from build123d import *

# Parameters (mm, degrees)
SKETCH_W        = 45
SKETCH_H        = 43
PAD_DEPTH       = 65
SKETCH001_W     = 42
SKETCH001_H     = 42
POCKET_DEPTH    = 37
POCKET001_DEPTH = 43.001
SKETCH003_R     = 12
SKETCH003_R_2   = 1.5
POCKET002_DEPTH = 28.001
SKETCH004_R     = 6
POCKET003_DEPTH = 10
SKETCH005_W     = 62
SKETCH005_H     = 40
SKETCH005_R     = 2
PAD001_DEPTH    = 2
FILLET_R        = 2


with BuildPart() as part:
    # Sketch → Pad (new body)
    with BuildSketch(Plane.YZ):
        with Locations((22.5, 21.5)):
            Rectangle(SKETCH_W, SKETCH_H)
    extrude(amount=PAD_DEPTH)

    # Sketch001 (on Face6 of Pad) → Pocket (cut)
    with BuildSketch(Plane.YZ.offset(65)):
        with Locations((22.5, 21.5)):
            Rectangle(SKETCH001_W, SKETCH001_H)
    extrude(amount=-POCKET_DEPTH, mode=Mode.SUBTRACT)

    # Sketch002 (on Face6 of Pocket) → Pocket001 (cut, through all)
    with BuildSketch(Plane(origin=(0, 0, 43), x_dir=(0, -1, 0), z_dir=(0, 0, 1))):
        Polygon((-43.5, 65), (0, 28), (0, 65), align=None)
    extrude(amount=-POCKET001_DEPTH, mode=Mode.SUBTRACT)

    # Sketch003 (on Face12 of Pocket001) → Pocket002 (cut, through all)
    with BuildSketch(Plane.YZ.offset(28)):
        with Locations((22.5, 21.5)):
            Circle(SKETCH003_R)
        with Locations((7, 37)):
            Circle(SKETCH003_R_2)
        with Locations((38, 37)):
            Circle(SKETCH003_R_2)
        with Locations((7, 6)):
            Circle(SKETCH003_R_2)
        with Locations((38, 6)):
            Circle(SKETCH003_R_2)
    extrude(amount=-POCKET002_DEPTH, mode=Mode.SUBTRACT)

    # Sketch004 (on Face1 of Pocket002) → Pocket003 (cut)
    with BuildSketch(Plane.YX):
        with Locations((15, 10)):
            Circle(SKETCH004_R)
    extrude(amount=-POCKET003_DEPTH, mode=Mode.SUBTRACT)

    # Sketch005 (on Face4 of Pocket003) → Pad001 (join)
    with BuildSketch(Plane.ZX.offset(45)):
        with Locations((21.5, 45)):
            Rectangle(SKETCH005_W, SKETCH005_H)
        with Locations((-5.5, 60)):
            Circle(SKETCH005_R, mode=Mode.SUBTRACT)
        with Locations((-5.5, 45)):
            Circle(SKETCH005_R, mode=Mode.SUBTRACT)
        with Locations((-5.5, 30)):
            Circle(SKETCH005_R, mode=Mode.SUBTRACT)
        with Locations((48.5, 60)):
            Circle(SKETCH005_R, mode=Mode.SUBTRACT)
        with Locations((48.5, 45)):
            Circle(SKETCH005_R, mode=Mode.SUBTRACT)
        with Locations((48.5, 30)):
            Circle(SKETCH005_R, mode=Mode.SUBTRACT)
    extrude(amount=PAD001_DEPTH)

    # Fillet
    fillet_edges = [part.edges().sort_by_distance(p)[0] for p in [
        (65, 46, 52.5),
        (25, 46, 52.5),
        (65, 46, -9.5),
        (25, 46, -9.5),
    ]]
    fillet(fillet_edges, radius=FILLET_R)


solid = part.part
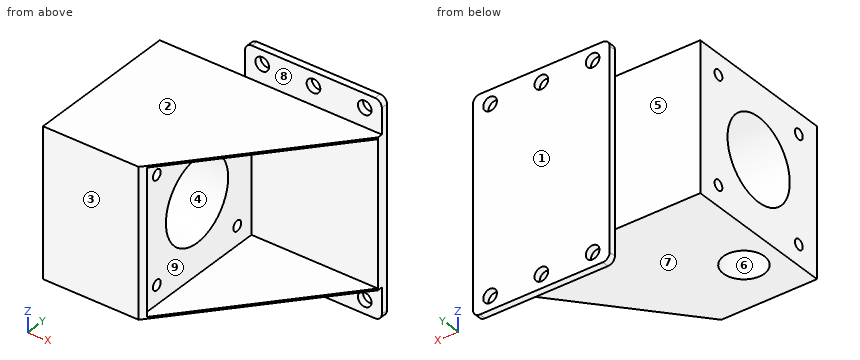
The listing builds one solid part. Answer for the finished solid, in the listing's coordinates (mm). Face numbers are marked on the shaded views. A direction names the side the tool comes from. Give positions to 0.01 mm unless a question says otherwise; leave off trailing zeros. Order: outer loops, then holes, each group sorted by start corner. A loop starts at its lowest first (then second) coordinate and runs counter-clockwise, first axis right, second up. Notation, with made-up numbers: (-11, 16.5) -> (12, 16.5) arc R19 cw to (12, 42.5) -> close; hole circle Ø9 at (70, 51). An arc over 180 degrees is marked (long way). Put each result on its own line as item: value.
Item 1: For a pull along Y with two mould halves and no side action, classify the marked faces 1, 2, 3 and 4 as released by +Y, released by -Y, zero draft, split by the parting line, or undercut.
Established:
face 1: released by +Y
face 2: zero draft
face 3: released by -Y
face 4: undercut
Item 2: Straight lines are drawn through the part: line 1 (Z direction, x = 6, y = 38); line 2 (X direction, y = 45.45, z = -5.5); line 3 (Y direction, x = 10, z = 8). For each, find the intervals that lie inside material, in ascending order.
Established:
line 1: z = 0 to 4.5, 7.5 to 35.5, 38.5 to 43
line 2: x = 25 to 28, 32 to 43, 47 to 58, 62 to 65
line 3: y = 0 to 9, 21 to 45
Item 3: Given P1, Ø2, axis at y = 46.5, z = 10, coming from the -X side; P2, Ø5, axis at y = 7, z = 37, coming from the +X side; P3, Ø5, axis at x = 39.5, z = -3.5, coming from the -Y side; P4, Ø2.5, axis at x = 30, z = 48.5, coming from the -Y side, each flat-ended and moving along its own axis, determine where each tip first touches the part or whether it passes through.
Established:
P1: stops at x = 25
P2: stops at x = 28
P3: stops at y = 45
P4: passes through
Item 4: A cutting plane is placed at A-A on z = 6. Give the vertices of the cut face in (x, y).
Established:
outline: (0, 0) -> (28, 0) -> (29.28, 1.5) -> (28, 1.5) -> (28, 5.5) -> (0, 5.5) -> close; (0, 8.5) -> (28, 8.5) -> (28, 36.5) -> (0, 36.5) -> close; (0, 39.5) -> (28, 39.5) -> (28, 43.5) -> (65, 43.5) -> (65, 47) -> (25, 47) -> (25, 45) -> (0, 45) -> close; hole circle Ø12 at (10, 15)
Item 5: A cutting plane is placed at C-C on z = 37. Give the vertices of the cut face in (x, y).
Established:
outline: (0, 0) -> (28, 0) -> (29.28, 1.5) -> (28, 1.5) -> (28, 5.5) -> (0, 5.5) -> close; (0, 8.5) -> (28, 8.5) -> (28, 36.5) -> (0, 36.5) -> close; (0, 39.5) -> (28, 39.5) -> (28, 43.5) -> (65, 43.5) -> (65, 47) -> (25, 47) -> (25, 45) -> (0, 45) -> close
Item 6: For the marked faces 5, 6, 7, 8 and 9, determine the directions among +Z, -Z, +X, -X, +Y, -Y from which every point of the face is accessible in a straight line to the end or side of a thin tool.
Established:
face 5: +Z, -Z, -X, +Y
face 6: -Z
face 7: -Z, +X, -X, -Y
face 8: +Z, +X, -X, -Y
face 9: +X
Item 7: A cutting plane is placed at D-D on y = 31.5. Give the vertices of the cut face in (x, z), plus the area to 3 significant figures.
Established:
outline: (0, 0) -> (54.79, 0) -> (54.79, 0.5) -> (28, 0.5) -> (28, 13.56) -> (0, 13.56) -> close; (0, 29.44) -> (28, 29.44) -> (28, 42.5) -> (54.79, 42.5) -> (54.79, 43) -> (0, 43) -> close
area: 786 mm^2
Item 8: A cutting plane is placed at B-B on z = -5.5. Give the vertices of the cut face in (x, y), plus the area to 3 significant figures.
Established:
outline: (25, 45) -> (28, 45) -> (28, 47) -> (25, 47) -> close; (32, 45) -> (43, 45) -> (43, 47) -> (32, 47) -> close; (47, 45) -> (58, 45) -> (58, 47) -> (47, 47) -> close; (62, 45) -> (65, 45) -> (65, 47) -> (62, 47) -> close
area: 56.0 mm^2
